Model file for the job. Use its own axes, mm. A direction names the side the tool comes from. Give positions to 0.01 mm unless a question says otherwise; leave off trailing zeros. Loops run counter-clockwise (first coordinate to the right, second up) from the corner with the lowest first, then second, coordinate; pieces in that order, holes last. Notation, with made-up numbers: M -36.5,-32.75 L 5.5,-32.75 A10 ccw 5.5,-22.75 Z; hole C 33,39 d9. An arc over 180 degrees is marked long. Answer in a Markdown table with one row per item.
```python
from build123d import *

# Parameters (mm, degrees)
SKETCH1_W           = 15.875
SKETCH1_H           = 69.85
BOSS_EXTRUDE1_DEPTH = 6.35
BOSS_EXTRUDE2_DEPTH = 6.35
BOSS_EXTRUDE3_DEPTH = 12.7
CUT_EXTRUDE1_DEPTH  = 41.411152545
CUT_EXTRUDE2_DEPTH  = 41.566760177


with BuildPart() as part:
    # Sketch1 → Boss-Extrude1 (new body)
    with BuildSketch(Plane(origin=(0, 0, 0), x_dir=(0, 0, -1), z_dir=(1, 0, 0))):
        Rectangle(SKETCH1_W, SKETCH1_H)
    extrude(amount=BOSS_EXTRUDE1_DEPTH)

    # Sketch2 → Boss-Extrude2 (add)
    with BuildSketch(Plane.ZY):
        Polygon((7.9375, 34.925), (-7.9375, 34.925), (-7.9375, 15.875), (7.9375, 18.674190819), align=None)
    extrude(amount=BOSS_EXTRUDE2_DEPTH)

    # Sketch3 → Boss-Extrude3 (add)
    with BuildSketch(Plane.ZY):
        Polygon((-7.9375, -19.944190819), (-7.9375, -34.925), (7.9375, -34.925), (7.9375, -17.145), align=None)
    extrude(amount=BOSS_EXTRUDE3_DEPTH)

    # Sketch6 → Cut-Extrude1 (cut, through all)
    with BuildSketch(Plane(origin=(0, 0, -7.9375), x_dir=(-1, 0, 0), z_dir=(0, 0, -1))):
        Polygon((0, -17.145), (12.7, -17.145), (12.7, -19.384352655), align=None)
    extrude(amount=-CUT_EXTRUDE1_DEPTH, mode=Mode.SUBTRACT)

    # Sketch7 → Cut-Extrude2 (cut, through all)
    with BuildSketch(Plane(origin=(6.35, 0, 0), x_dir=(0, 0, -1), z_dir=(1, 0, 0))):
        with BuildLine():
            Line((3.5687, 28.841737989), (3.5687, 23.761737989))
            ThreePointArc((3.5687, 23.761737989), (0, 20.193037989), (-3.5687, 23.761737989))
            Line((-3.5687, 23.761737989), (-3.5687, 28.841737989))
            ThreePointArc((-3.5687, 28.841737989), (0, 32.410437989), (3.5687, 28.841737989))
        make_face()
    extrude(amount=-CUT_EXTRUDE2_DEPTH, mode=Mode.SUBTRACT)


solid = part.part
```
Q1. Probe probe 1 along Y at (x, z) = (-2.75, 2.25) (3 decimals); probe 2 along Y at (x, z) = (-4.25, 1) (3 decimals); probe 3 along X at (y, z) = (-4, 2.75). List the from-to ranges inside material, lowest first.
Reported:
| item | result |
|---|---|
| probe 1 | -34.925 to -18.148, 17.671 to 20.992, 31.612 to 34.925 |
| probe 2 | -34.925 to -18.368, 17.451 to 20.336, 32.267 to 34.925 |
| probe 3 | 0 to 6.35 |
Q2. Drop a flat-ended pin along its axis: pin 1 (5 mm diameter, centred on y = 23, z = -3.5, fed in from -X). Give the stop position or say it passes through.
Reported:
| item | result |
|---|---|
| pin 1 | x = -6.35 |
Q3. 3-axis set-ups, long thin cutter, end or side, ignore diameter. For faces 5 (the face through (-4.85, -18.836, -1.653)), 6 (the face through (-3.131, 17.255, -0.111)), 7 (the face through (-6.35, 26, -4)), 8 (the face through (0.089, 20.194, -0.078)), 9 (the face through (-12.7, -27, 0)): which of +Z, -Z, +X, -X, +Y, -Y reach the whole face in a straight line?
Reported:
| item | result |
|---|---|
| face 5 | -Z, -X |
| face 6 | +Z, -X |
| face 7 | +Z, -Z, -X, +Y |
| face 8 | +X, -X |
| face 9 | +Z, -Z, -X, +Y, -Y |
Q4. Saw through at B-B (y = 26). Give the cut face in (x, z).
Reported:
| item | result |
|---|---|
| outline | M -6.35,-7.94 L 6.35,-7.94 L 6.35,-3.57 L -6.35,-3.57 Z; M -6.35,3.57 L 6.35,3.57 L 6.35,7.94 L -6.35,7.94 Z |
Q5. Saw through at D-D (x = -5.25). Give the cut face in (y, z) (1 decimal), and give its area (3 significant figures).
Reported:
| item | result |
|---|---|
| outline | M -34.9,-7.9 L -19.9,-7.9 L -18.1,2.7 L -18.1,7.9 L -34.9,7.9 Z; M 15.9,-7.9 L 34.9,-7.9 L 34.9,7.9 L 18.7,7.9 Z; hole M 23.8,-3.6 L 28.8,-3.6 A3.6 ccw 28.8,3.6 L 23.8,3.6 A3.6 ccw Z |
| area | 462 mm² |
Q6. Saw through at A-A (x = 2.5). Give the cut face in (y, z) (1 decimal), and give its area (3 significant figures).
Reported:
| item | result |
|---|---|
| outline | M -34.9,-7.9 L 34.9,-7.9 L 34.9,7.9 L -34.9,7.9 Z; hole M 23.8,-3.6 L 28.8,-3.6 A3.6 ccw 28.8,3.6 L 23.8,3.6 A3.6 ccw Z |
| area | 1,030 mm² |
Q7. Mould opens along Y. For faces 1 (the face through (-3, -34.925, 0)), 2 (the face through (0, 26, -3.569)), 3 (the face through (1, 0, -7.938)), 4 (the face through (-9.261, -18.778, 4.321)) say: released by +Y, released by -Y, zero draft, split by the parting line, or undercut.
Reported:
| item | result |
|---|---|
| face 1 | released by -Y |
| face 2 | undercut |
| face 3 | zero draft |
| face 4 | undercut |
